Verification items for this drawing (mm, ordinates from the low corner). A direction names the side the tool comes from. Round coordinates to 2 decimals unless told otherwise and drop trailing zeros. Order: outer loops, then holes, each group sorted by start corner. A loop starts at its lowest first (then second) coordinate and runs counter-clockwise, first axis right, second up. Notation, with made-up numbers: M 73.5,51 L 97.5,51 A28 ccw 97.5,88 Z; hole C 34,79.5 d8. An arc over 180 degrees is marked long. Use CSV: the item, a comma, the result in double quotes. Start each with the question number.
Q1. Scan lines: line 1 (Y direction, x = 145.5, z = 3.65); line 2 (Y direction, x = 90.5, z = 8.1); line 3 (Y direction, x = 89.5, z = 1.5). Record each from-to range of solid material in increasing order.
Q2. Sectioned sample at A-A (y = 9.5). Enter the section's corners in (x, z).
Q3. Set-up check for the marked faces 1 and 2: record each of +Z, -Z, +X, -X, +Y, -Y from which the full face is reachable in a straight line by a thin tool's end or side.
Q4. Gauge pin test, flat end, axial feed: pin 1 Ø1 at (x, y) = (79.5, 36) entering from +Z. Record the tip position at first contact, or that the pin passes through.
Q5. Sectioned sample at D-D (x = 77). Enter the section's corners in (y, z), and give its area (3 significant figures).
Q6. Sectioned sample at B-B (x = 145.5). Enter the section's corners in (y, z).
Q7. Sectioned sample at C-C (y = 44). Enter the section's corners in (x, z), and give its area (3 significant figures).
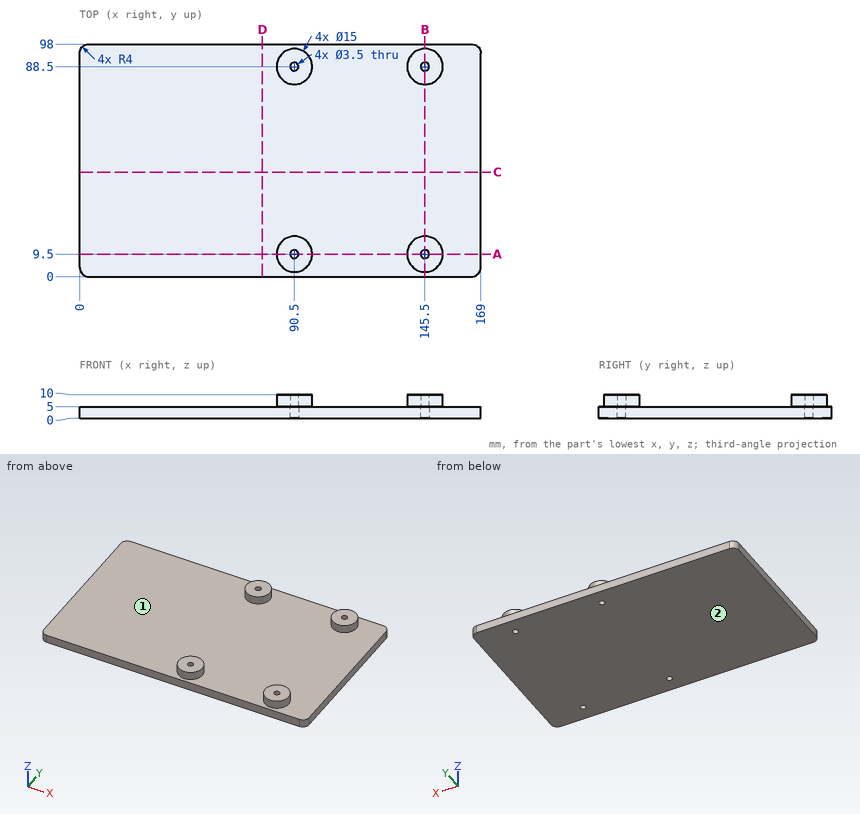
Verdict:
1,line 1,"y = 0 to 7.75, 11.25 to 86.75, 90.25 to 98"
1,line 2,"y = 2 to 7.75, 11.25 to 17, 81 to 86.75, 90.25 to 96"
1,line 3,"y = 0 to 8.06, 10.94 to 87.06, 89.94 to 98"
2,outline,"M 0,0 L 88.75,0 L 88.75,10 L 83,10 L 83,5 L 0,5 Z; M 92.25,0 L 143.75,0 L 143.75,10 L 138,10 L 138,5 L 98,5 L 98,10 L 92.25,10 Z; M 147.25,0 L 169,0 L 169,5 L 153,5 L 153,10 L 147.25,10 Z"
3,face 1,"+Z"
3,face 2,"-Z, +X, -X, +Y, -Y"
4,pin 1,"stops at z = 5"
5,outline,"M 0,0 L 98,0 L 98,5 L 0,5 Z"
5,area,"490 mm²"
6,outline,"M 0,0 L 7.75,0 L 7.75,10 L 2,10 L 2,5 L 0,5 Z; M 11.25,0 L 86.75,0 L 86.75,10 L 81,10 L 81,5 L 17,5 L 17,10 L 11.25,10 Z; M 90.25,0 L 98,0 L 98,5 L 96,5 L 96,10 L 90.25,10 Z"
7,outline,"M 0,0 L 169,0 L 169,5 L 0,5 Z"
7,area,"845 mm²"
